```python
from build123d import *

# Parameters (mm, degrees)
BOSS_EXTRUDE1_DEPTH = 368.3
SKETCH2_R           = 2.032
CUT_EXTRUDE1_DEPTH  = 25.4


with BuildPart() as part:
    # Sketch1 → Boss-Extrude1 (new body)
    with BuildSketch(Plane(origin=(0, 0, 0), x_dir=(1, 0, 0), z_dir=(0, 1, 0))):
        Polygon((0, 0), (3.175, 0), (3.175, 22.225), (22.225, 22.225), (22.225, 0), (25.4, 0), (25.4, 25.4), (0, 25.4), align=None)
    extrude(amount=BOSS_EXTRUDE1_DEPTH)

    # Sketch2 → Cut-Extrude1 (cut)
    with BuildSketch(Plane.ZY):
        with Locations((-12.7, 71.4375)):
            Circle(SKETCH2_R)
        with Locations((-12.7, 296.8625)):
            Circle(SKETCH2_R)
        with Locations((-12.7, 287.3375)):
            Circle(SKETCH2_R)
        with Locations((-12.7, 80.9625)):
            Circle(SKETCH2_R)
    extrude(amount=-CUT_EXTRUDE1_DEPTH, mode=Mode.SUBTRACT)


solid = part.part
```
Check sheet for the modelled part. Datum: model origin and axes. Units: mm. A direction names the side the tool comes from. Give positions to 0.01 mm unless a question says otherwise; leave off trailing zeros. Order: outer loops, then holes, each group sorted by start corner. A loop starts at its lowest first (then second) coordinate and runs counter-clockwise, first axis right, second up. Notation, with made-up numbers: M 28.5,48.5 L 51.5,48.5 A26 cw 51.5,65.5 Z; hole C -14.75,6 d3. An arc over 180 degrees is marked long. Answer in a Markdown table with one row per item. Add a question column.
Q1. Access from +Z, -Z, +X, -X, +Y, -Y to the whole of each face (thin tool, end or side, straight path). Record for faces 4 (the flat face through (3.175, 182, -11)), 5 (the flat face through (12, 0, -23)).
Q2. Sectioned sample at C-C, the plane x = 13.75. Record the boundary of the cut face in (y, z) (3 decimals), and give its area (3 significant figures).
Q3. Gauge pin test, flat end, axial feed: pin 1 Ø12 at (x, z) = (7, -7.5) entering from +Y. Record the tip position at first contact, or that the pin passes through.
Q4. Release check for a two-part mould opening along X. For faces 1 (the flat face through (13, 182, -22.225)), 2 (the flat face through (25.4, 182, -13)), 3 (the flat face through (13, 182, -25.4)) record: released by +X, released by -X, zero draft, split by the parting line, or undercut.
Q5. Thickness scan on L1, parallel to Y at x = 1.2, z = -12.7; L2, parallel to X at y = 88.5, z = -14.25 (3 decimals); L3, parallel to Z at x = 7, y = 165 (3 decimals). Record the ranges inside material, lowest first.
Q6. Sectioned sample at A-A, the plane z = -3.75. Record the boundary of the cut face in (x, y) (3 decimals).
Q7. Sectioned sample at B-B, the plane y = 170. Record the boundary of the cut face in (x, z) (3 decimals).
Verdict:
| question | item | result |
|---|---|---|
| 1 | face 4 | +Z, +Y, -Y |
| 1 | face 5 | +Z, -Z, +X, -X, -Y |
| 2 | outline | M 0,-25.4 L 368.3,-25.4 L 368.3,-22.225 L 0,-22.225 Z |
| 2 | area | 1,170 mm² |
| 3 | pin 1 | y = 368.3 |
| 4 | face 1 | undercut |
| 4 | face 2 | released by +X |
| 4 | face 3 | zero draft |
| 5 | L1 | 0 to 69.41, 73.47 to 78.93, 82.99 to 285.31, 289.37 to 294.83, 298.89 to 368.3 |
| 5 | L2 | 0 to 3.175, 22.225 to 25.4 |
| 5 | L3 | -25.4 to -22.225 |
| 6 | outline | M 0,0 L 3.175,0 L 3.175,368.3 L 0,368.3 Z; M 22.225,0 L 25.4,0 L 25.4,368.3 L 22.225,368.3 Z |
| 7 | outline | M 0,-25.4 L 25.4,-25.4 L 25.4,0 L 22.225,0 L 22.225,-22.225 L 3.175,-22.225 L 3.175,0 L 0,0 Z |
